Part model, mm, in its own coordinate system. A direction names the side the tool comes from. Round coordinates to 2 decimals unless told otherwise and drop trailing zeros. Write each loop counter-clockwise with the first axis right and the second up, starting at its lowest first coordinate (ties: lowest second). Pieces come first, ordered by that corner, then holes. Notation, with made-up numbers: M -23.75,14.25 L 31.25,14.25 A14 ccw 31.25,21.25 Z; hole C 43,1 d5. An arc over 180 degrees is marked long. Use one line per item in the form item = value. Start each with the question number.
Item 1: Probe L1, parallel to Y at x = -114, z = -2; L2, parallel to Z at x = -32, y = 2.5; L3, parallel to Z at x = 4, y = 13. List the from-to ranges inside material, lowest first.
Item 2: Cut at C-C, the plane y = 16.5. Give the cut face in (x, z), then the cut area to 3 significant figures.
Item 3: Mould opens along Y. For faces 1 (the face through (-83.381, 26.085, -2.465)), 2 (the face through (-2, 25, -5)), 3 (the face through (-125.189, 39.437, -1.479)) say: +Y half, -Y half, draft (parallel to the pull), parting line (faces both ways), or undercut.
Item 4: Cut at B-B, the plane x = 83.5. Give the cut face in (y, z), then the cut area to 3 significant figures.
Item 5: Which spindle directions (+Z, -Z, +X, -X, +Y, -Y) get a long thin tool onto all of the face, cutting with end or side? Do faces 4 (the face through (31, 2, -24)), 5 (the face through (7, 28, -2)), 6 (the face through (-30, 5, -11)). Say none if no direction does.
Item 6: Flat gauge pins, fed straight in: pin 1 Ø11.5 at (x, y) = (-88, 28) entering from -Z; pin 2 Ø10 at (y, z) = (36, -4) entering from +X; pin 3 Ø8 at (x, y) = (-114, 28) entering from -Z; pin 4 Ø18.5 at (x, z) = (25, -18.5) entering from +Y. Where does each tip first touch, or does it go through?
Item 7: Cut at A-A, the plane x = -7.5. Give the cut face in (y, z), then the cut area to 3 significant figures.
from build123d import *

# Parameters (mm, degrees)
F1_DEPTH = 5
F2_R     = 5
F3_DEPTH = 5
F4_W     = 260
F4_H     = 5
F5_DEPTH = 27
F6_R     = 14
F8_DEPTH = 5
F9_R     = 2


with BuildPart() as f1:
    # F0 (on Top) → F1 (new body)
    with BuildSketch(Plane.XY):
        with BuildLine():
            Line((-130, 0), (130, 0))
            Line((130, 0), (130, 28))
            ThreePointArc((130, 28), (125.313708, 39.313708), (114, 44))
            Line((114, 44), (-114, 44))
            ThreePointArc((-114, 44), (-125.313708, 39.313708), (-130, 28))
            Line((-130, 28), (-130, 0))
        make_face()
    extrude(amount=-F1_DEPTH)

    # F2 (on face) → F3 (cut)
    with BuildSketch(Plane.XY):
        with BuildLine():
            Line((12, 23), (114, 23))
            ThreePointArc((114, 23), (119, 28), (114, 33))
            Line((114, 33), (12, 33))
            ThreePointArc((12, 33), (7, 28), (12, 23))
        make_face()
        with Locations((-88, 28)):
            Circle(F2_R)
        with Locations((-114, 28)):
            Circle(F2_R)
    extrude(amount=-F3_DEPTH, mode=Mode.SUBTRACT)

    # F4 (on face) → F5 (join)
    with BuildSketch(Plane(origin=(0, 0, -5), x_dir=(1, 0, 0), z_dir=(0, 0, -1))):
        with Locations((0, -2.5)):
            Rectangle(F4_W, F4_H)
    extrude(amount=F5_DEPTH)

    # F6
    f6_edges = [f1.edges().sort_by_distance(p)[0] for p in [
        (130, 2.5, -32),
        (-130, 2.5, -32),
    ]]
    fillet(f6_edges, radius=F6_R)

    # F7 (on face) → F8 (cut)
    with BuildSketch(Plane.XZ):
        with BuildLine():
            ThreePointArc((112, -24), (118, -18), (112, -12))
            Line((112, -12), (-48, -12))
            ThreePointArc((-48, -12), (-54, -18), (-48, -24))
            Line((-48, -24), (112, -24))
        make_face()
    extrude(amount=-F8_DEPTH, mode=Mode.SUBTRACT)

    # F9
    f9_edges = [f1.edges().sort_by_distance(p)[0] for p in [
        (0, 5, -32),
        (0, 44, -5),
        (0, 5, -5),
    ]]
    fillet(f9_edges, radius=F9_R)


solid = f1.part
Model answer:
q1.L1 = 0 to 23, 33 to 44
q1.L2 = -32 to -24, -12 to 0
q1.L3 = -5 to 0
q2.outline = M -130,-3 A2 ccw -128,-5 L 128,-5 A2 ccw 130,-3 L 130,0 L -130,0 Z
q2.area = 1,300 mm²
q3.face_1 = undercut
q3.face_2 = draft
q3.face_3 = +Y half
q4.outline = M 0,-32 L 3,-32 A2 ccw 5,-30 L 5,-24 L 0,-24 Z; M 0,-12 L 5,-12 L 5,-7 A2 cw 7,-5 L 23,-5 L 23,0 L 0,0 Z; M 33,-5 L 42,-5 A2 ccw 44,-3 L 44,0 L 33,0 Z
q4.area = 244 mm²
q5.face_4 = +Y, -Y
q5.face_5 = +Z, -Z
q5.face_6 = -Z, +X, -X, +Y
q6.pin_1 = -5
q6.pin_2 = 129.7
q6.pin_3 = through
q6.pin_4 = 5
q7.outline = M 0,-32 L 3,-32 A2 ccw 5,-30 L 5,-24 L 0,-24 Z; M 0,-12 L 5,-12 L 5,-7 A2 cw 7,-5 L 42,-5 A2 ccw 44,-3 L 44,0 L 0,0 Z
q7.area = 294 mm²
